Part model, mm, in its own coordinate system. Face numbers are marked on the shaded views. Coordinates: 2 decimals unless noted, no trailing zeros. Write each loop counter-clockwise with the first axis right and the second up, starting at its lowest first coordinate (ties: lowest second). Pieces come first, ordered by that corner, then holes. Notation, with made-up numbers: (13.25, 41.5) - (67.25, 41.5) arc R37 ccw to (67.25, 80.5) - close; hole circle Ø10 at (-3, -6). An arc over 180 degrees is marked (long way). Use a Markdown table: item, result.
```python
from build123d import *

# Parameters (mm, degrees)
MAIN_BODY_DEPTH                  = 3.81
CROSS_SCREW_BOSSES_DEPTH         = 31.75
F_8_CLEARANCE_HOLE1_D            = 4.4958
BALLOON_MONOFILAMENT_HOLE_D      = 2.5273
PARACHUTE_MONOFILAMENT_HOLE_D    = 2.5273
SKETCH21_W                       = 12.08
SKETCH21_H                       = 11.74
HOT_WIRE_CUTTER_HOLDER_DEPTH     = 9.67
CUT_EXTRUDE10_START              = -1.27
CUT_EXTRUDE10_DEPTH              = 63.383576094
CHAMFER8_SIZE                    = 0.381
SKETCH22_W                       = 6.029522694
SKETCH22_H                       = 1.524
SATELLITE_CABLE_MANAGEMENT_DEPTH = 66.050272386


with BuildPart() as part:
    # Sketch3 → Main body (new body)
    with BuildSketch(Plane.XY):
        with BuildLine():
            Line((-15.875, -38.1), (-15.875, 38.1))
            ThreePointArc((-15.875, 38.1), (-18.260491841, 42.291797068), (-23.082694008, 42.38179842))
            ThreePointArc((-23.082694008, 42.38179842), (-28.900226452, 38.649767283), (-34.12497326, 34.12497326))
            ThreePointArc((-34.12497326, 34.12497326), (-35.921024484, 34.12497326), (-35.921024484, 35.921024484))
            ThreePointArc((-35.921024484, 35.921024484), (0, 50.8), (35.921024484, 35.921024484))
            ThreePointArc((35.921024484, 35.921024484), (35.921024484, 34.12497326), (34.12497326, 34.12497326))
            ThreePointArc((34.12497326, 34.12497326), (28.900226452, 38.649767283), (23.082694008, 42.38179842))
            ThreePointArc((23.082694008, 42.38179842), (18.260491841, 42.291797068), (15.875, 38.1))
            Line((15.875, 38.1), (15.875, -38.1))
            ThreePointArc((15.875, -38.1), (18.260491841, -42.291797068), (23.082694008, -42.38179842))
            ThreePointArc((23.082694008, -42.38179842), (28.900226452, -38.649767283), (34.12497326, -34.12497326))
            ThreePointArc((34.12497326, -34.12497326), (35.921024484, -34.12497326), (35.921024484, -35.921024484))
            ThreePointArc((35.921024484, -35.921024484), (0, -50.8), (-35.921024484, -35.921024484))
            ThreePointArc((-35.921024484, -35.921024484), (-35.921024484, -34.12497326), (-34.12497326, -34.12497326))
            ThreePointArc((-34.12497326, -34.12497326), (-28.900226452, -38.649767283), (-23.082694008, -42.38179842))
            ThreePointArc((-23.082694008, -42.38179842), (-18.260491841, -42.291797068), (-15.875, -38.1))
        make_face()
    extrude(amount=MAIN_BODY_DEPTH)

    # Sketch5 → Cross screw bosses (add)
    with BuildSketch(Plane(origin=(15.875, 0, 0), x_dir=(0, 0, -1), z_dir=(1, 0, 0))):
        with BuildLine():
            Line((0, 38.1), (0, 26.99385))
            Line((0, 26.99385), (0, 14.29385))
            ThreePointArc((0, 14.29385), (1.86498297, 18.77886703), (6.35, 20.64385))
            ThreePointArc((6.35, 20.64385), (12.699998494, 26.998224058), (6.341251887, 33.343843974))
            ThreePointArc((6.341251887, 33.343843974), (2.338844583, 34.612930799), (0, 38.1))
        make_face()
        with BuildLine():
            ThreePointArc((6.261703048, -20.644463916), (1.864650947, -18.840779739), (0, -14.469233029))
            Line((0, -14.469233029), (0, -26.99385))
            Line((0, -26.99385), (0, -38.1))
            ThreePointArc((0, -38.1), (2.217611083, -34.670801888), (6.077775616, -33.338012189))
            ThreePointArc((6.077775616, -33.338012189), (6.213919542, -33.33945129), (6.35, -33.34385))
            ThreePointArc((6.35, -33.34385), (12.7, -26.99385), (6.35, -20.64385))
            ThreePointArc((6.35, -20.64385), (6.305852606, -20.644312569), (6.261703048, -20.644463916))
        make_face()
    extrude(amount=-CROSS_SCREW_BOSSES_DEPTH)

    # 8 Clearance Hole1 (through all)
    with Locations(Plane(origin=(15.875, 0, 0), x_dir=(0, 0, -1), z_dir=(1, 0, 0))):
        with Locations((6.35, 26.99385), (6.35, -26.893399733)):
            Hole(F_8_CLEARANCE_HOLE1_D / 2)

    # Balloon monofilament hole (through all)
    with Locations(Plane.XY.offset(3.81)):
        with Locations((-9.525, 0)):
            Hole(BALLOON_MONOFILAMENT_HOLE_D / 2)

    # Parachute monofilament hole (through all)
    with Locations(Plane.XY.offset(3.81)):
        with Locations((9.525, 0)):
            Hole(PARACHUTE_MONOFILAMENT_HOLE_D / 2)

    # Sketch21 → Hot wire cutter holder (add)
    with BuildSketch(Plane.XY.offset(-8.5979)):
        with Locations((-5.315, -27.056)):
            Rectangle(SKETCH21_W, SKETCH21_H)
    extrude(amount=-HOT_WIRE_CUTTER_HOLDER_DEPTH)

    # Sketch21_10 → Cut-Extrude10 (cut, through all)
    with BuildSketch(Plane.XY.offset(-8.5979).offset(CUT_EXTRUDE10_START)):
        with BuildLine():
            Line((-4.243, -30.386), (-2.315, -30.386))
            ThreePointArc((-2.315, -30.386), (-1.961446609, -30.239553391), (-1.815, -29.886))
            Line((-1.815, -29.886), (-1.815, -24.786))
            Line((-1.815, -24.786), (-1.765, -24.786))
            ThreePointArc((-1.765, -24.786), (-1.623578644, -24.727421356), (-1.565, -24.586))
            Line((-1.565, -24.586), (-1.565, -24.386))
            Line((-1.565, -24.386), (-1.815, -24.386))
            Line((-1.815, -24.386), (-1.815, -21.186))
            Line((-1.815, -21.186), (-8.815, -21.186))
            Line((-8.815, -21.186), (-8.815, -30.386))
            Line((-8.815, -30.386), (-7.418, -30.386))
            Line((-7.418, -30.386), (-7.418, -32.926))
            Line((-7.418, -32.926), (-4.243, -32.926))
            Line((-4.243, -32.926), (-4.243, -30.386))
        make_face()
    extrude(amount=-CUT_EXTRUDE10_DEPTH, mode=Mode.SUBTRACT)

    # Chamfer8
    chamfer8_edges = [part.edges().sort_by_distance(p)[0] for p in [
        (-8.1165, -30.386, -18.2679),
        (-8.815, -25.786, -18.2679),
        (-3.279, -30.386, -18.2679),
        (-1.961446609, -30.239553391, -18.2679),
        (-1.815, -27.336, -18.2679),
    ]]
    chamfer(chamfer8_edges, length=CHAMFER8_SIZE)

    # Sketch22 → satellite cable management (cut, through all)
    with BuildSketch(Plane(origin=(0, 0, 0), x_dir=(-1, 0, 0), z_dir=(0, 0, -1))):
        with Locations((0, -47.038383029)):
            Rectangle(SKETCH22_W, SKETCH22_H)
        with Locations((0, -41.958383029)):
            Rectangle(SKETCH22_W, SKETCH22_H)
    extrude(amount=-SATELLITE_CABLE_MANAGEMENT_DEPTH, mode=Mode.SUBTRACT)


solid = part.part
```
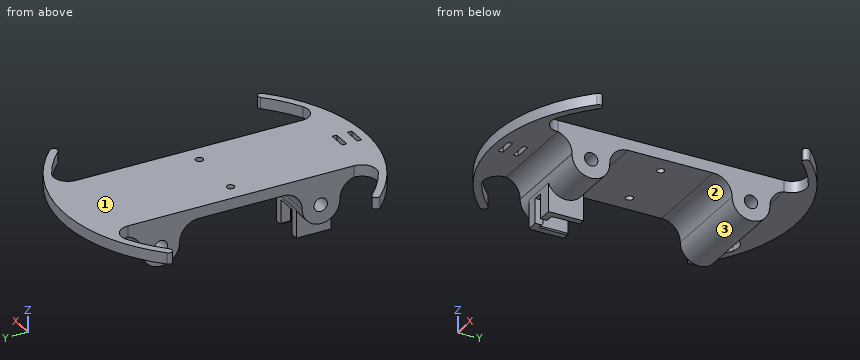
Item 1: Drill centre lines: probe 1 along Y at (x, z) = (-0.5, 2.25); probe 2 along Y at (x, z) = (4, -6.35); probe 3 along Y at (x, z) = (-9, -13.25). Where is each one in solid material? Low to high.
From the geometry:
| item | result |
|---|---|
| probe 1 | -50.8 to -47.8, -46.28 to -42.72, -41.2 to 50.8 |
| probe 2 | -33.34 to -29.14, -24.65 to -20.64, 20.64 to 24.75, 29.24 to 33.34 |
| probe 3 | -32.93 to -21.19 |
Item 2: Drop flat-ended pins along their axis: P1, Ø10, axis at x = -17.5, y = -36.5, coming from the -Z side; P2, Ø0.8, axis at y = -47.5, z = 2, coming from the -X side; P3, Ø1.7, axis at y = -42, z = 2, coming from the +X side; P4, Ø8, axis at x = -4, y = -26, coming from the -Z side. Give the stop position or say it passes through.
From the geometry:
| item | result |
|---|---|
| P1 | z = -10.53 |
| P2 | x = -19.03 |
| P3 | x = 29.79 |
| P4 | z = -18.27 |
Item 3: Band-saw the part on D-D, the plane x = 28. Give the cut face in (y, z).
From the geometry:
| item | result |
|---|---|
| outline | (-42.39, 0) - (-39.31, 0) - (-39.31, 3.81) - (-42.39, 3.81) - close; (39.31, 0) - (42.39, 0) - (42.39, 3.81) - (39.31, 3.81) - close |
Item 4: Band-saw the part on B-B, the plane y = 0. Give the cut face in (x, z) (3 decimals).
From the geometry:
| item | result |
|---|---|
| outline | (-15.875, 0) - (-10.789, 0) - (-10.789, 3.81) - (-15.875, 3.81) - close; (-8.261, 0) - (8.261, 0) - (8.261, 3.81) - (-8.261, 3.81) - close; (10.789, 0) - (15.875, 0) - (15.875, 3.81) - (10.789, 3.81) - close |
Item 5: Band-saw the part on A-A, the plane z = -15.5. Give the cut face in (x, y) (3 decimals).
From the geometry:
| item | result |
|---|---|
| outline | (-11.355, -32.926) - (-7.418, -32.926) - (-7.418, -30.386) - (-8.815, -30.386) - (-8.815, -21.186) - (-11.355, -21.186) - close; (-4.243, -32.926) - (0.725, -32.926) - (0.725, -21.186) - (-1.815, -21.186) - (-1.815, -24.386) - (-1.565, -24.386) - (-1.565, -24.586) arc R0.2 cw to (-1.765, -24.786) - (-1.815, -24.786) - (-1.815, -29.886) arc R0.5 cw to (-2.315, -30.386) - (-4.243, -30.386) - close |
Item 6: Band-saw the part on C-C, the plane z = 2.75. Give the cut face in (x, y) (3 decimals), then the cut area to 3 significant figures.
From the geometry:
| item | result |
|---|---|
| outline | (-35.921, -35.921) arc R50.8 ccw to (35.921, -35.921) arc R1.27 ccw to (34.125, -34.125) arc R48.26 cw to (23.083, -42.382) arc R4.876 cw to (15.875, -38.1) - (15.875, 38.1) arc R4.876 cw to (23.083, 42.382) arc R48.26 cw to (34.125, 34.125) arc R1.27 ccw to (35.921, 35.921) arc R50.8 ccw to (-35.921, 35.921) arc R1.27 ccw to (-34.125, 34.125) arc R48.26 cw to (-23.083, 42.382) arc R4.876 cw to (-15.875, 38.1) - (-15.875, -38.1) arc R4.876 cw to (-23.083, -42.382) arc R48.26 cw to (-34.125, -34.125) arc R1.27 ccw to start; hole circle Ø2.527 at (-9.525, 0); hole (-3.015, -47.8) - (3.015, -47.8) - (3.015, -46.276) - (-3.015, -46.276) - close; hole (-3.015, -42.72) - (3.015, -42.72) - (3.015, -41.196) - (-3.015, -41.196) - close; hole circle Ø2.527 at (9.525, 0) |
| area | 3,440 mm^2 |
Item 7: Two-plate mould, pull along Y, no slides. Class the marked faces 1, 2 and 3: pulls with the +Y half, pulls with the -Y half, needs draft (parallel to the pull), parting line crosses it, or undercut.
From the geometry:
| item | result |
|---|---|
| face 1 | needs draft |
| face 2 | undercut |
| face 3 | undercut |
